from build123d import *

# Parameters (mm, degrees)
SKETCH003_W = 16
SKETCH003_H = 16
SKETCH004_W = 14
SKETCH004_H = 14
SKETCH_W    = 14.5
SKETCH_H    = 14.1
SKETCH005_W = 12.7
SKETCH005_H = 13.1
SKETCH006_W = 1
SKETCH006_H = 3
PAD_DEPTH   = 4
FILLET_R    = 2
FILLET001_R = 1
FILLET002_R = 0.5


with BuildPart() as part:
    # Sketch003 → AdditiveLoft section 0
    with BuildSketch(Plane.XY):
        Rectangle(SKETCH003_W, SKETCH003_H)
    # Sketch004 → AdditiveLoft section 1
    with BuildSketch(Plane(origin=(0, 0, 5.8), x_dir=(1, 0, 0), z_dir=(0, -0.087156, 0.996195))):
        Rectangle(SKETCH004_W, SKETCH004_H)
    loft()

    # Sketch (on Face1 of AdditiveLoft) → SubtractiveLoft section 0
    with BuildSketch(Plane(origin=(0, 0, 0), x_dir=(1, 0, 0), z_dir=(0, 0, -1))):
        Rectangle(SKETCH_W, SKETCH_H)
    # Sketch005 → SubtractiveLoft section 1
    with BuildSketch(Plane.XY.offset(3.1)):
        Rectangle(SKETCH005_W, SKETCH005_H)
    loft(mode=Mode.SUBTRACT)

    # Sketch006 (on Face11 of SubtractiveLoft) → Pad (new body)
    with BuildSketch(Plane(origin=(0, 0, 3.1), x_dir=(1, 0, 0), z_dir=(0, 0, -1))):
        with Locations((-2.7, 0)):
            Rectangle(SKETCH006_W, SKETCH006_H)
    pad = extrude(amount=PAD_DEPTH)

    # Mirrored: Pad across Sketch006 V_Axis
    add(pad.mirror(Plane(origin=(0, 0, 3.1), x_dir=(0, 0, -1), z_dir=(1, 0, 0))))

    # Fillet
    fillet_edges = [part.edges().sort_by_distance(p)[0] for p in [
        (-7.5, -7.486681, 2.594955),
        (-7.5, 7.486681, 3.205045),
        (7.5, 7.486681, 3.205045),
        (7.5, -7.486681, 2.594955),
    ]]
    fillet(fillet_edges, radius=FILLET_R)

    # Fillet001
    fillet001_edges = [part.edges().sort_by_distance(p)[0] for p in [
        (-6.8, -6.8, 1.55),
        (-6.8, 6.8, 1.55),
        (6.8, -6.8, 1.55),
        (6.8, 6.8, 1.55),
    ]]
    fillet(fillet001_edges, radius=FILLET001_R)

    # Fillet002
    fillet002_edges = [part.edges().sort_by_distance(p)[0] for p in [
        (-3.2, 0, 3.1),
        (2.2, 0, 3.1),
        (-2.7, -1.5, 3.1),
        (2.7, -1.5, 3.1),
        (3.2, 0, 3.1),
        (-2.2, 0, 3.1),
        (2.7, 1.5, 3.1),
        (-2.7, 1.5, 3.1),
    ]]
    fillet(fillet002_edges, radius=FILLET002_R)


solid = part.part
Input: part model. Units: mm. Frame: model coordinates. A direction names the side the tool comes from. Give positions to 0.01 mm unless a question says otherwise; leave off trailing zeros. Use CSV: the item, a comma, the result in double quotes. Start each with the question number.
Item 1: Reachability of faces 1 (the flat face through (-3, 1.5, 1)), 2 (the flat face through (3, 0, -0.9)) from +Z, -Z, +X, -X, +Y, -Y: full face, straight path, thin tool, end or side. Return the list, or none.
Item 2: Mould query, pull axis Y, two halves, no side actions, for faces 3 (the flat face through (-0.2, 0, 5.8)), 4 (the flat face through (-2.2, 0, 1)), 5 (the flat face through (-0.6, -7.2, 0)). Classes: pulls with the +Y half, pulls with the -Y half, needs draft (parallel to the pull), parting line crosses it, or undercut.
Item 3: Line query: line 1 (X direction, y = -0.25, z = 2); line 2 (Y direction, x = 3, z = 1.5); line 3 (X direction, y = 0, z = -0.5). Output: solid intervals per line, ascending.
Item 4: Section A-A on z = 2. State how many separate pieces and enclosed holes the cut face has, then the cut area to 3 significant figures.
Item 5: Contact query for flat-ended pins moving along their axis: P1, Ø1.5, axis at y = 0, z = 1, coming from the +X side; P2, Ø1.5, axis at x = -4, z = 4.5, coming from the -Y side; P3, Ø0.9, axis at y = 0.5, z = 1.5, coming from the +X side. Output: stop coordinate, or through.
Ans:
1,face 1,"-Z"
1,face 2,"-Z, +X, -X, +Y, -Y"
2,face 3,"pulls with the -Y half"
2,face 4,"undercut"
2,face 5,"needs draft"
3,line 1,"x = -7.65 to -6.67, -3.2 to -2.2, 2.2 to 3.2, 6.67 to 7.65"
3,line 2,"y = -7.7 to -6.81, -1.5 to 1.5, 6.81 to 7.76"
3,line 3,"x = -3.2 to -2.2, 2.2 to 3.2"
4,separate pieces,"3"
4,enclosed holes,"1"
4,area,"58.0 mm2"
5,P1,"stops at x = 7.96"
5,P2,"stops at y = -7.26"
5,P3,"stops at x = 7.82"
